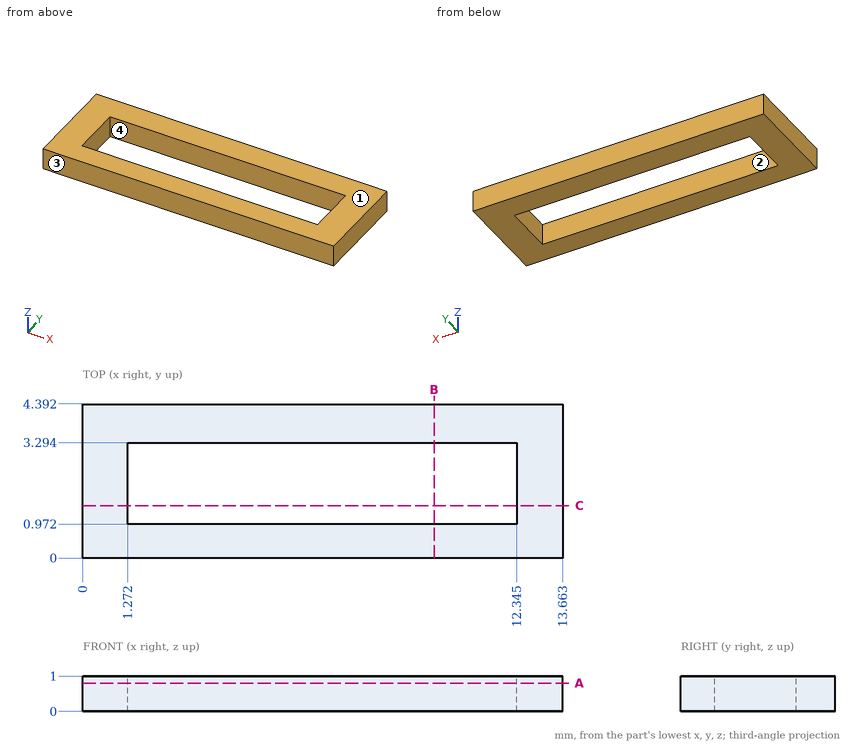
Geometry check sheet. Reference: drawing and pictorial views, mm from the part's lowest x, y, z. A direction names the side the tool comes from. Coordinates: 2 decimals unless noted, no trailing zeros. Loops run counter-clockwise (first coordinate to the right, second up) from the corner with the lowest first, then second, coordinate; pieces in that order, holes last. Notation, with made-up numbers: (-40, 57.25) -> (11, 57.25) arc R21 ccw to (11, 89.25) -> close; hole circle Ø9 at (-30.5, -22.75). An arc over 180 degrees is marked (long way). Put each result on its own line as item: value.
1) Thickness scan on line 1 (Y direction, x = 10.5, z = 0.5); line 2 (X direction, y = 1.1, z = 0.2) (1 decimal). Record the ranges inside material, lowest first.
Result set:
line 1: y = 0 to 0.97, 3.29 to 4.39
line 2: x = 0 to 1.3, 12.3 to 13.7
2) Cross-section at B-B on x = 10. Record the boundary of the cut face in (y, z).
Result set:
outline: (0, 0) -> (0.97, 0) -> (0.97, 1) -> (0, 1) -> close; (3.29, 0) -> (4.39, 0) -> (4.39, 1) -> (3.29, 1) -> close
3) Cross-section at A-A on z = 0.8. Record the boundary of the cut face in (x, y) (1 decimal).
Result set:
outline: (0, 0) -> (13.7, 0) -> (13.7, 4.4) -> (0, 4.4) -> close; hole (1.3, 1) -> (12.3, 1) -> (12.3, 3.3) -> (1.3, 3.3) -> close
4) Release check for a two-part mould opening along X. For the marked faces 3 and 4 record: released by +X, released by -X, zero draft, split by the parting line, or undercut.
Result set:
face 3: zero draft
face 4: undercut
5) Cross-section at C-C on y = 1.5. Record the boundary of the cut face in (x, z) (1 decimal).
Result set:
outline: (0, 0) -> (1.3, 0) -> (1.3, 1) -> (0, 1) -> close; (12.3, 0) -> (13.7, 0) -> (13.7, 1) -> (12.3, 1) -> close
6) Tool access check on the marked faces 1 and 2. Record the directions out of +Z, -Z, +X, -X, +Y, -Y that give a thin tool (end or side, any length) a straight path to the whole face; none if there is none.
Result set:
face 1: +Z, +X, -X, +Y, -Y
face 2: +Z, -Z
